Autodesk Inventor part; units mm, degrees
ref_plane "YZ Plane" through (0, 0, 0) normal (1, 0, 0) x (0, 1, 0)
ref_plane "XZ Plane" through (0, 0, 0) normal (0, 1, 0) x (-1, 0, 0)
ref_plane "XY Plane" through (0, 0, 0) normal (0, 0, 1) x (1, 0, 0)
sketch "Skizze1" plane through (0, 0, 0) normal (0, 1, 0) x (-1, 0, 0)
  line L0 (-32.5, 30) -> (32.5, 30)
  line L1 (32.5, 30) -> (32.5, -30)
  line L2 (32.5, -30) -> (-32.5, -30)
  line L3 (-32.5, -30) -> (-32.5, 30)
  line L4 (-32.5, 30) -> (32.5, -30) construction
  line L5 (32.5, 30) -> (-32.5, -30) construction
  point P0 (0, 0)
  dimension "d0" = 65
  dimension "d1" = 60
extrude "Extrusion1" add sketch "Skizze1" along normal blind 7
sketch "Skizze2" plane through (0, 7, 0) normal (0, 1, 0) x (1, 0, 0)
  line L0 (24.5, -20) -> (-24.5, -20)
  line L1 (-24.5, -20) -> (-24.5, 20)
  line L2 (-24.5, 20) -> (24.5, 20)
  line L3 (24.5, 20) -> (24.5, -20)
  line L4 (24.5, -20) -> (-24.5, 20) construction
  line L5 (-24.5, -20) -> (24.5, 20) construction
  line L6 (29.8936, 0) -> (-30.3656, 0) construction
  point P0 (0, 0)
  point P1 (0, 0)
  point P2 (-24.5, 0)
  point P3 (24.5, 0)
  dimension "d4" = 49
  dimension "d5" = 40
hole "Bohrung1" [suppressed]
sketch "Skizze3" plane through (0, 0, 0) normal (0, -1, 0) x (1, 0, 0)
  line L0 (-18, -18) -> (18, -18)
  line L1 (18, -18) -> (18, 18)
  line L2 (18, 18) -> (-18, 18)
  line L3 (-18, 18) -> (-18, -18)
  line L4 (-18, -18) -> (18, 18) construction
  line L5 (18, -18) -> (-18, 18) construction
  line L6 (0, -22.3415) -> (0, 25.3309) construction
  point P0 (0, 0)
  point P1 (0, 18)
  point P2 (0, -18)
  dimension "d13" = 36
  dimension "d14" = 36
hole "Bohrung2" at (0, 0, 18) at (0, 0, -18) at (-18, 0, 18) at (-18, 0, -18) at (18, 0, 18) at (18, 0, -18) direction (0, 1, 0) diameter 3.4 depth 8 tip angle 118 counterbore diameter 6.5 counterbore depth 3.4
sketch "Skizze4" plane through (0, 0, 0) normal (0, -1, 0) x (1, 0, 0)
  circle A0 centre (18, 18) radius 3.25
  circle A1 centre (-18, 18) radius 3.25
  circle A2 centre (0, 18) radius 3.25
  circle A3 centre (0, -18) radius 3.25
  circle A4 centre (-18, -18) radius 3.25
  circle A5 centre (18, -18) radius 3.25
  line L0 (32.5, 30) -> (-32.5, 30)
  line L1 (-32.5, 30) -> (-32.5, -30)
  line L2 (-32.5, -30) -> (32.5, -30)
  line L3 (32.5, -30) -> (32.5, 30)
  line L4 (-32.5, 30) -> (-27, 30)
  line L5 (-27, 30) -> (-27, -30)
  line L6 (-27, -30) -> (-32.5, -30)
  line L7 (-32.5, -30) -> (-32.5, 30)
  line L8 (32.5, -30) -> (-32.5, -30)
  line L9 (27, -30) -> (32.5, -30)
  line L10 (32.5, -30) -> (32.5, 30)
  line L11 (32.5, 30) -> (27, 30)
  line L12 (27, 30) -> (27, -30)
  point P0 (0, 0)
  dimension "d22" = 54
  dimension "d23" = 65
  dimension "d24" = 5.5
extrude "Extrusion2" add sketch "Skizze4" along normal blind 10 contours L3 L2 L12 L0 | L5 L2 L1 L0
sketch "Skizze5" plane through (-32.5, 7, -30) normal (-1, 0, 0) x (0, 0, 1)
  line L0 (0, -7) -> (60, -7)
  line L1 (0, -7) -> (0, -17)
  line L2 (60, -17) -> (0, -17)
  line L3 (60, -7) -> (60, -17)
  point P0 (30, -7)
  point P1 (35, -12)
  dimension "d27" = 5
  dimension "d41" = 35
  dimension "d42" = 60
hole "Bohrung3" at (-32.5, -5, 5) direction (1, 0, 0) diameter 3.4 end through all
pattern_linear "Rechteckige Anordnung1" count 3 spacing 20 along (0, 0, -1) of "Bohrung3" first direction both ways yes
chamfer "Fase2" distance 10 angle 45 2 edges at (-29.75, -10, -30) (29.75, -10, -30)
chamfer "Fase3" distance 4 angle 45 2 edges at (-29.75, -10, 30) (29.75, -10, 30)
equation "\"d24\" = -0.5 * d22 + 0.5 * d23"
properties part number "complex_cube_plane" material "Aluminium 6061"
Model file for the job. Use its own axes, mm. A direction names the side the tool comes from. Give positions to 0.01 mm unless a question says otherwise; leave off trailing zeros. Write each loop counter-clockwise with the first axis right and the second up, starting at its lowest first coordinate (ties: lowest second). Pieces come first, ordered by that corner, then holes. Notation, with made-up numbers: (14, -23) -> (34, -23) arc R30 cw to (34, 10) -> close; hole circle Ø2 at (-16.5, 63.5). An arc over 180 degrees is marked (long way). Write item = value, one per line.
(1) Flat gauge pins, fed straight in: P1, Ø3, axis at x = 1.5, z = -19.5, coming from the -Y side; P2, Ø6, axis at x = -18, z = 18, coming from the -Y side. Where does each tip first touch, or does it go through?
Determined:
P1 = 0
P2 = 3.4
(2) Slice it at A-A, the plane y = -8.25. Give the cut face in (x, z), then the cut area to 4 significant figures.
Determined:
outline = (-32.5, -21.75) -> (-27, -21.75) -> (-27, 27.75) -> (-32.5, 27.75) -> close; (27, -21.75) -> (32.5, -21.75) -> (32.5, 27.75) -> (27, 27.75) -> close
area = 544.5 mm2
(3) Probe line 1 along Z through (x, y) = (-18, 2); line 2 along X through (y, z) = (4.65, -18); line 3 along Z through (x, y) = (-18, 5.65). List the from-to ranges inside material, lowest first.
Determined:
line_1 = -30 to -21.25, -14.75 to 14.75, 21.25 to 30
line_2 = -32.5 to -19.7, -16.3 to -1.7, 1.7 to 16.3, 19.7 to 32.5
line_3 = -30 to -19.7, -16.3 to 16.3, 19.7 to 30
(4) Slice it at B-B, the plane x = 18. Give the cut face in (y, z).
Determined:
outline = (0, -30) -> (7, -30) -> (7, -19.7) -> (3.4, -19.7) -> (3.4, -21.25) -> (0, -21.25) -> close; (0, -14.75) -> (3.4, -14.75) -> (3.4, -16.3) -> (7, -16.3) -> (7, 16.3) -> (3.4, 16.3) -> (3.4, 14.75) -> (0, 14.75) -> close; (0, 21.25) -> (3.4, 21.25) -> (3.4, 19.7) -> (7, 19.7) -> (7, 30) -> (0, 30) -> close
(5) Tool access for faces 5 (the face through (27, -5, 0)), 6 (the face through (-18.143, 1.724, 21.247)), 7 (the face through (0, 3, -30)): list every direction of +Z, -Z, +X, -X, +Y, -Y with a clear straight run to the whole face (end or side of a thin tool).
Determined:
face_5 = +Z, -Z, -Y
face_6 = -Y
face_7 = -Z, +X, -X, +Y, -Y
(6) Mould opens along X. For faces 1 (the face through (29.79, -4.35, 26.57)), 2 (the face through (-32.5, -2, 0)), 3 (the face through (-0.143, 1.724, 21.247)), 4 (the face through (18.65, 5.23, 16.43)) say: released by +X, released by -X, zero draft, split by the parting line, or undercut.
Determined:
face_1 = zero draft
face_2 = released by -X
face_3 = undercut
face_4 = undercut
(7) Slice it at C-C, the plane z = 25. Give the cut face in (x, y).
Determined:
outline = (-32.5, -10) -> (-27, -10) -> (-27, -6.7) -> (-32.5, -6.7) -> close; (-32.5, -3.3) -> (-27, -3.3) -> (-27, 0) -> (27, 0) -> (27, -3.3) -> (32.5, -3.3) -> (32.5, 7) -> (-32.5, 7) -> close; (27, -10) -> (32.5, -10) -> (32.5, -6.7) -> (27, -6.7) -> close
(8) Slice it at D-D, the plane y = -5. Give the number of separate pieces and of enclosed holes in the cut face, then the cut area to 3 significant figures.
Determined:
separate_pieces = 8
enclosed_holes = 0
area = 493 mm2
